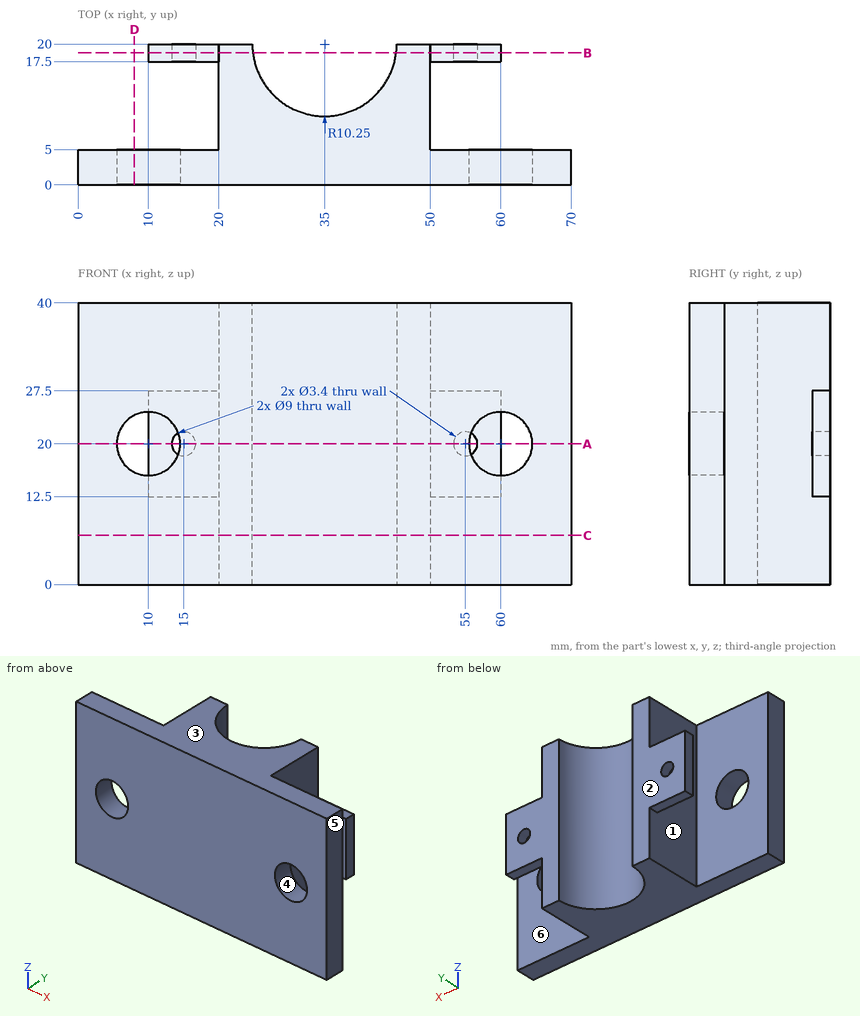
Check sheet for the drawn part. Datum: minimum x, y, z corner. Units: mm. A direction names the side the tool comes from. Round coordinates to 2 decimals unless told otherwise and drop trailing zeros. Write each loop counter-clockwise with the first axis right and the second up, starting at its lowest first coordinate (ties: lowest second). Pieces come first, ordered by that corner, then holes. Notation, with made-up numbers: (58.5, -16.75) -> (67.5, -16.75) arc R8 ccw to (67.5, -1.75) -> close; hole circle Ø3 at (80.25, -3.5). An arc over 180 degrees is marked (long way). Write each question's results on one line, items separated by ' | '.
Q1. Sectioned sample at D-D, the plane x = 8. Record the boundary of the cut face in (y, z).
Derived:
outline: (0, 0) -> (5, 0) -> (5, 15.97) -> (0, 15.97) -> close; (0, 24.03) -> (5, 24.03) -> (5, 40) -> (0, 40) -> close
Q2. Access from +Z, -Z, +X, -X, +Y, -Y to the whole of each face (thin tool, end or side, straight path). Record for the marked faces 4, 5 and 6.
Derived:
face 4: -Y | face 5: +Z, -Z, +X, +Y, -Y | face 6: +Z, -Z, +X
Q3. Sectioned sample at B-B, the plane y = 18.75. Record the boundary of the cut face in (x, z).
Derived:
outline: (10, 12.5) -> (20, 12.5) -> (20, 0) -> (24.83, 0) -> (24.83, 40) -> (20, 40) -> (20, 27.5) -> (10, 27.5) -> close; (45.17, 0) -> (50, 0) -> (50, 12.5) -> (60, 12.5) -> (60, 27.5) -> (50, 27.5) -> (50, 40) -> (45.17, 40) -> close; hole circle Ø3.4 at (15, 20); hole circle Ø3.4 at (55, 20)
Q4. Go/stop test with flat-tipped pins: pin 1 Ø5 at (y, z) = (6.5, 27) entering from +X; pin 2 Ø10 at (x, y) = (59.5, 13.5) entering from -Z; pin 3 Ø8 at (x, z) = (60, 20) entering from -Y; pin 4 Ø3 at (x, y) = (15, 19) entering from +Z. Record where each tip stops, or that it passes through.
Derived:
pin 1: stops at x = 70 | pin 2: stops at z = 12.5 | pin 3: stops at y = 17.5 | pin 4: stops at z = 27.5
Q5. Sectioned sample at A-A, the plane z = 20. Give the number of separate pieces and of enclosed holes in the cut face, and give its area (3 significant figures).
Derived:
separate pieces: 5 | enclosed holes: 0 | area: 578 mm²
Q6. Thickness scan on probe 1 along X at (y, z) = (1.75, 18.5); probe 2 along Y at (x, z) = (55.5, 11); probe 3 along X at (y, z) = (14.25, 32.5). Record the ranges inside material, lowest first.
Derived:
probe 1: x = 0 to 5.76, 14.24 to 55.76, 64.24 to 70 | probe 2: y = 0 to 5 | probe 3: x = 20 to 26.51, 43.49 to 50
Q7. Sectioned sample at C-C, the plane z = 7. Record the boundary of the cut face in (x, y), and give its area (3 significant figures).
Derived:
outline: (0, 0) -> (70, 0) -> (70, 5) -> (50, 5) -> (50, 20) -> (45.25, 20) arc R10.25 cw to (24.75, 20) -> (20, 20) -> (20, 5) -> (0, 5) -> close | area: 635 mm²
Q8. Draft check along Y on the marked faces 1, 2 and 3. Enter one of: released by +Y, released by -Y, zero draft, split by the parting line, or undercut.
Derived:
face 1: undercut | face 2: released by +Y | face 3: zero draft
